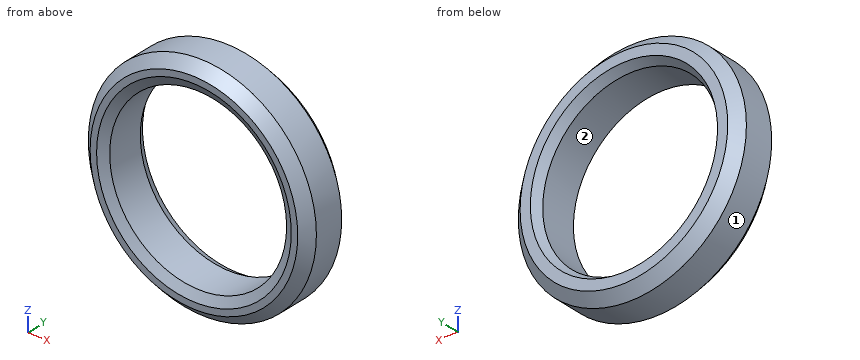
from build123d import *

# Parameters (mm, degrees)
SKETCH1_R             = 11.15
SKETCH1_R_2           = 8.65
BOSS_EXTRUDE1_DEPTH   = 5
CHAMFER1_SIZE         = 1
CHAMFER2_SIZE         = 0.5
CHAMFER2_SIZE2        = 0.866025404
CHAMFER2_PART_2_SIZE  = 0.5
CHAMFER2_PART_2_SIZE2 = 0.866025404


with BuildPart() as part:
    # Sketch1 → Boss-Extrude1 (new body)
    with BuildSketch(Plane(origin=(0, 0, 0), x_dir=(1, 0, 0), z_dir=(0, 1, 0))):
        Circle(SKETCH1_R)
        Circle(SKETCH1_R_2, mode=Mode.SUBTRACT)
    extrude(amount=BOSS_EXTRUDE1_DEPTH)

    # Chamfer1
    chamfer1_edges = [part.edges().sort_by_distance(p)[0] for p in [
        (-11.15, 0, 0),
        (-11.15, 5, 0),
    ]]
    chamfer(chamfer1_edges, length=CHAMFER1_SIZE)

    # Chamfer2
    chamfer2_edges = [part.edges().sort_by_distance(p)[0] for p in [
        (-8.65, 0, 0),
    ]]
    chamfer2_side = [part.faces().sort_by_distance(p)[0] for p in [
        (-8.65, 2.5, 0),
    ]]
    chamfer(chamfer2_edges, length=CHAMFER2_SIZE, length2=CHAMFER2_SIZE2, reference=chamfer2_side[0])

    # Chamfer2 part 2
    chamfer2_part_2_edges = [part.edges().sort_by_distance(p)[0] for p in [
        (-8.65, 5, 0),
    ]]
    chamfer2_part_2_side = [part.faces().sort_by_distance(p)[0] for p in [
        (-9.862914647, 5, 0),
    ]]
    chamfer(chamfer2_part_2_edges, length=CHAMFER2_PART_2_SIZE, length2=CHAMFER2_PART_2_SIZE2, reference=chamfer2_part_2_side[0])


solid = part.part
Geometry check sheet. Reference: the model listing, model coordinates, mm. Face numbers are marked on the shaded views. Round coordinates to 2 decimals unless told otherwise and drop trailing zeros. Order: outer loops, then holes, each group sorted by start corner. A loop starts at its lowest first (then second) coordinate and runs counter-clockwise, first axis right, second up. Notation, with made-up numbers: M -26,87 L 23,87 A11 ccw 23,108 Z; hole C 67.5,79 d5. An arc over 180 degrees is marked long. Answer in a Markdown table with one row per item. Add a question column.
Item 1: Depth check by flat-ended pin: pin 1 Ø1.5 at (y, z) = (2.5, -2.5) entering from -X; pin 2 Ø1.5 at (y, z) = (4, -4) entering from +X; pin 3 Ø3 at (y, z) = (2, -8) entering from +X. Enter the tip coordinate at first touch or a pass-through.
Item 2: Sectioned sample at A-A, the plane z = 0. Enter the section's corners in (x, y), plus the area to 3 significant figures.
Item 3: Sectioned sample at B-B, the plane x = 0. Enter the section's corners in (y, z), plus the area to 3 significant figures.
Item 4: Sectioned sample at C-C, the plane y = 3.4. Enter the section's corners in (x, z).
Item 5: Draft check along Z on the marked faces 1 and 2. Enter one of: released by +Z, released by -Z, zero draft, split by the parting line, or undercut.
Item 6: Material ranges on L1, parallel to X at y = 2.6, z = 0; L2, parallel to X at y = 1.6, z = -6.75, recorded low to high. Write a range as [from, to].
Filled in:
| question | item | result |
|---|---|---|
| 1 | pin 1 | stops at x = -11.01 |
| 1 | pin 2 | stops at x = 10.67 |
| 1 | pin 3 | stops at x = 9.06 |
| 2 | outline | M -11.15,1 L -10.15,0 L -9.52,0 L -8.65,0.5 L -8.65,4.13 L -9.15,5 L -10.15,5 L -11.15,4 Z; M 8.65,0.5 L 9.52,0 L 10.15,0 L 11.15,1 L 11.15,4 L 10.15,5 L 9.15,5 L 8.65,4.13 Z |
| 2 | area | 22.1 mm² |
| 3 | outline | M 0,-10.15 L 1,-11.15 L 4,-11.15 L 5,-10.15 L 5,-9.15 L 4.13,-8.65 L 0.5,-8.65 L 0,-9.52 Z; M 0,9.52 L 0.5,8.65 L 4.13,8.65 L 5,9.15 L 5,10.15 L 4,11.15 L 1,11.15 L 0,10.15 Z |
| 3 | area | 22.1 mm² |
| 4 | outline | C 0,0 d22.3; hole C 0,0 d17.3 |
| 5 | face 1 | split by the parting line |
| 5 | face 2 | undercut |
| 6 | L1 | x = [-11.15, -8.65], [8.65, 11.15] |
| 6 | L2 | x = [-8.87, -5.41], [5.41, 8.87] |
